CAD build for the part. Positions are in the model's coordinates, mm. Face numbers are marked on the shaded views. A direction names the side the tool comes from. Coordinates: 2 decimals unless noted, no trailing zeros. Loops run counter-clockwise (first coordinate to the right, second up) from the corner with the lowest first, then second, coordinate; pieces in that order, holes last.
1) Saw through at B-B, the plane z = -189.5. Write the cut outline in (x, y), and give its area (3 significant figures).
2) Which spindle directions (+Z, -Z, +X, -X, +Y, -Y) get a long thin tool onto all of the face, cutting with end or side? Do the marked faces 5, 6 and 7. Say none if no direction does.
3) Two-plate mould, pull along Y, no slides. Class the marked faces 1, 2, 3 and 4: +Y half, -Y half, draft (parallel to the pull), parting line (faces both ways), or undercut.
4) Saw through at C-C, the plane y = 138. Write the cut outline in (x, z).
5) Wall check: line 1 along Z through (x, y) = (15, 2.8); line 2 along X through (y, z) = (1.85, -40); line 3 along Y through (x, z) = (196, -85.5). Give the ranges that are in metal, low to high.
6) Pin check, flat tips, straight feed: pin 1 Ø6 at (x, y) = (144.5, 47) entering from -Z; pin 2 Ø2 at (y, z) = (70, -51) entering from +X; pin 3 Ø8 at (x, z) = (425, -175) entering from +Y. Stop position of each tip, or through.
Autodesk Inventor part; units mm, degrees
ref_plane "YZ Plane" through (0, 0, 0) normal (1, 0, 0) x (0, 1, 0)
ref_plane "XZ Plane" through (0, 0, 0) normal (0, 1, 0) x (-1, 0, 0)
ref_plane "XY Plane" through (0, 0, 0) normal (0, 0, 1) x (1, 0, 0)
sketch "Sketch1" plane through (0, 0, 0) normal (0, 0, 1) x (1, 0, 0)
  line L0 (0, 0) -> (440, 0)
  line L1 (220, 0) -> (380, 0)
  line L2 (220, 0) -> (60, 0)
  line L3 (60, 2.9881) -> (60, 155)
  line L4 (60, 155) -> (380, 155)
  line L5 (380, 155) -> (380, 0)
  line L6 (60, -5) -> (220, -5)
  line L7 (220, -5) -> (385, -5)
  line L8 (385, -5) -> (385, 160)
  line L9 (385, 160) -> (55, 160)
  line L10 (55, 160) -> (55, 2.9881)
  line L11 (0, 0) -> (0, 5)
  line L12 (0, 5) -> (440, 5)
  line L13 (440, 5) -> (440, 0)
  point P0 (385, 5)
  point P1 (55, 5)
  point P2 (380, 5)
  point P3 (60, 5)
  dimension "d0" = 440
  dimension "d1" = 160
  dimension "d2" = 160
  dimension "d4" = 5
  dimension "d5" = 5
  dimension "d16" = 150
extrude "Extrusion1" add sketch "Sketch1" against normal blind 215 contours L11 L12 L5 L0 | L10 L9 L8 L12 L5 L4 L3 | L5 L12 L8 L0 | L8 L12 L13 L0
sketch "Sketch2" plane through (0, 5, 0) normal (0, 1, 0) x (1, 0, 0)
  line L0 (0, 0) -> (0, 215)
  line L1 (0, 215) -> (15, 215)
  line L2 (440, 215) -> (0, 215)
  line L3 (15, 215) -> (15, -133.1496)
  line L4 (440, 215) -> (425, 215)
  line L5 (425, 215) -> (425, -133.1496)
  circle A0 centre (15, 175) radius 2.5
  circle A1 centre (15, 40) radius 2.5
  line L6 (55, 0) -> (0, 0)
  line L7 (220, 215) -> (220, -93.5309)
  circle A2 centre (425, 175) radius 2.5
  circle A3 centre (425, 40) radius 2.5
  dimension "d8" = 15
  dimension "d9" = 15
  dimension "d10" = 5
  dimension "d11" = 5
  dimension "d12" = 40
  dimension "d13" = 40
extrude "Extrusion2" cut sketch "Sketch2" against normal blind 215 contours A3 L5 | L5 A3 | A2 L5 | L5 A2 | A1 L3 | L3 A1 | A0 L3 | L3 A0
sketch "Sketch3" plane through (0, 0, 0) normal (0, 0, 1) x (1, 0, 0)
  line L0 (0, 5) -> (55, 5)
  line L1 (55, 160) -> (385, 160)
  line L2 (55, 5) -> (385, 5)
  line L3 (385, 5) -> (385, 160)
  line L4 (385, 160) -> (55, 160)
  line L5 (55, 160) -> (55, 5)
  point P0 (0, 0)
extrude "Extrusion3" add sketch "Sketch3" along normal blind 5
properties part number "Proteção de acrilico"
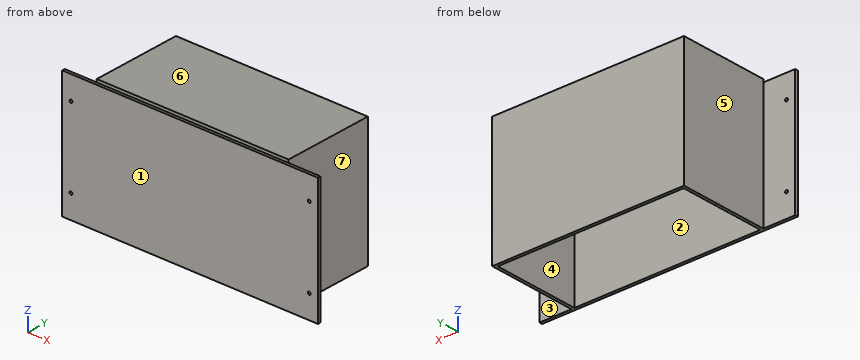
Data:
1. outline: (0, 0) - (440, 0) - (440, 5) - (385, 5) - (385, 160) - (55, 160) - (55, 5) - (0, 5) - close; hole (60, 5) - (380, 5) - (380, 155) - (60, 155) - close
1. area: 5,350 mm2
2. face 5: +Z, -Z, -X, +Y
2. face 6: +Z, +X, -X, +Y, -Y
2. face 7: +Z, -Z, +X, +Y
3. face 1: -Y half
3. face 2: undercut
3. face 3: +Y half
3. face 4: undercut
4. outline: (55, -215) - (60, -215) - (60, 0) - (380, 0) - (380, -215) - (385, -215) - (385, 5) - (55, 5) - close
5. line 1: z = -215 to -177.5, -172.5 to -42.5, -37.5 to 0
5. line 2: x = 0 to 12.5, 17.5 to 422.5, 427.5 to 440
5. line 3: y = 0 to 5, 155 to 160
6. pin 1: stops at z = 0
6. pin 2: stops at x = 385
6. pin 3: stops at y = 5
